Geometry: final body of the model. Coordinates: model frame, mm. A direction names the side the tool comes from. Round coordinates to 2 decimals unless told otherwise and drop trailing zeros. Write each loop counter-clockwise with the first axis right and the second up, starting at its lowest first coordinate (ties: lowest second). Pieces come first, ordered by that corner, then holes. Notation, with made-up numbers: (49, 13.25) -> (57, 13.25) arc R15 cw to (57, 28.25) -> close; hole circle Ø4 at (-15.5, -39). An arc over 180 degrees is marked (long way). One line per item, written item: value. Start each with the question number.
from build123d import *

# Parameters (mm, degrees)
BOSS_EXTRUDE1_DEPTH = 1219.2
SKETCH2_R           = 7.9375
CUT_EXTRUDE1_DEPTH  = 51.8
SKETCH4_R           = 3.96875
CUT_EXTRUDE3_DEPTH  = 44.45
LPATTERN1_COUNT     = 5
LPATTERN1_PITCH     = 203.2


with BuildPart() as part:
    # Sketch1 → Boss-Extrude1 (new body)
    with BuildSketch(Plane.XY):
        Polygon((0, 0), (-50.8, 0), (-50.8, -3.175), (-3.175, -3.175), (-3.175, -50.8), (0, -50.8), align=None)
    extrude(amount=BOSS_EXTRUDE1_DEPTH)

    # Sketch2 → Cut-Extrude1 (cut, through all)
    with BuildSketch(Plane(origin=(0, 0, 0), x_dir=(1, 0, 0), z_dir=(0, 1, 0))):
        with Locations((-38.1, -36.5125)):
            Circle(SKETCH2_R)
        with Locations((-38.1, -1182.6875)):
            Circle(SKETCH2_R)
        with Locations((-38.1, -152.4)):
            Circle(SKETCH2_R)
        with Locations((-38.1, -609.6)):
            Circle(SKETCH2_R)
        with Locations((-38.1, -990.6)):
            Circle(SKETCH2_R)
    extrude(amount=-CUT_EXTRUDE1_DEPTH, mode=Mode.SUBTRACT)

    # Sketch4 → Cut-Extrude3 (cut)
    with BuildSketch(Plane(origin=(-2.029899632, 0, 893.163272881), x_dir=(1, 0, 0), z_dir=(0, 1, 0))):
        with Locations((-39.245100368, 689.963272881)):
            Circle(SKETCH4_R)
    cut_extrude3 = extrude(amount=-CUT_EXTRUDE3_DEPTH, mode=Mode.SUBTRACT)

    # LPattern1: Cut-Extrude3 ×5, 1 skipped
    with Locations(*[(0, 0, i * LPATTERN1_PITCH) for i in range(1, LPATTERN1_COUNT) if i not in (2,)]):
        add(cut_extrude3, mode=Mode.SUBTRACT)


solid = part.part
(1) Section query A-A (z = 907.5). Output: boundary loops of the cut face in (x, y) (3 decimals).
(2) Line query: probe 1 along X at (y, z) = (-2.3, 609.6); probe 2 along X at (y, z) = (-10, 57) (3 decimals). Output: solid intervals per line, ascending.
(3) Section query B-B (y = -11.5). Output: boundary loops of the cut face in (x, z) (3 decimals).
(4) Set-up query: faces 1 (the face through (0, -26, 601)), 2 (the face through (-27, -3.175, 601)). Return all of +Z, -Z, +X, -X, +Y, -Y with unobstructed straight access to the full face (end or side cutting, diameter ignored); none if empty.
(5) Pin query (flat end, axial travel): pin 1 (20.5 mm diameter, centred on x = -38.1, z = 152.4, fed in from +Y); pin 2 (9.5 mm diameter, centred on x = -38.1, z = 36.51, fed in from +Y); pin 3 (5 mm diameter, centred on x = -42.5, z = 300.5, fed in from -Y) (3 decimals). Return the tip coordinate at first contact, or that it passes through.
Results list:
1. outline: (-50.8, -3.175) -> (-3.175, -3.175) -> (-3.175, -50.8) -> (0, -50.8) -> (0, 0) -> (-50.8, 0) -> close
2. probe 1: x = -50.8 to -46.04, -30.16 to 0
2. probe 2: x = -3.175 to 0
3. outline: (-3.175, 0) -> (0, 0) -> (0, 1219.2) -> (-3.175, 1219.2) -> close
4. face 1: +Z, -Z, +X, +Y, -Y
4. face 2: +Z, -Z, -X, -Y
5. pin 1: stops at y = 0
5. pin 2: passes through
5. pin 3: stops at y = -3.175
